from build123d import *

# Parameters (mm, degrees)
EXT_LUG_DEPTH = 2.4892


with BuildPart() as part:
    # Sk_kingpin_section → Rev_kingpin (revolve)
    with BuildSketch(Plane.XY, mode=Mode.PRIVATE) as rev_kingpin_sk:
        with BuildLine():
            Line((0, 54.2544), (5.9944, 52.64912))
            Line((5.9944, 52.64912), (5.9944, 45.12818))
            Line((5.9944, 45.12818), (6.49478, 44.6278))
            Line((6.49478, 44.6278), (6.93928, 44.6278))
            Line((6.93928, 44.6278), (7.43839, 45.12818))
            Line((7.43839, 45.12818), (7.43839, 60.1218))
            ThreePointArc((7.43839, 60.1218), (7.549982316, 60.391207684), (7.81939, 60.5028))
            Line((7.81939, 60.5028), (9.1567, 60.5028))
            ThreePointArc((9.1567, 60.5028), (9.426107684, 60.614392316), (9.5377, 60.8838))
            Line((9.5377, 60.8838), (9.5377, 63.1698))
            ThreePointArc((9.5377, 63.1698), (9.426107684, 63.439207684), (9.1567, 63.5508))
            Line((9.1567, 63.5508), (7.9121, 63.5508))
            ThreePointArc((7.9121, 63.5508), (7.642692316, 63.662392316), (7.5311, 63.9318))
            Line((7.5311, 63.9318), (7.5311, 69.34962))
            Line((7.5311, 69.34962), (7.03072, 69.85))
            Line((7.03072, 69.85), (0, 69.85))
            Line((0, 69.85), (0, 54.2544))
        make_face()
    revolve(rev_kingpin_sk.sketch.rotate(Axis((0, -25.4, 0), (0, 1, 0)), 90), axis=Axis((0, -25.4, 0), (0, 1, 0)))

    # Sk_lug → Ext_lug (add)
    with BuildSketch(Plane(origin=(0, 63.5508, 0), x_dir=(1, 0, 0), z_dir=(0, 1, 0))):
        with BuildLine():
            Line((-7.19328, 2.23012), (-7.19328, -2.23012))
            ThreePointArc((-7.19328, -2.23012), (-7.46394509, -1.797883422), (-7.9121, -1.55448))
            ThreePointArc((-7.9121, -1.55448), (-9.1313, 0), (-7.9121, 1.55448))
            ThreePointArc((-7.9121, 1.55448), (-7.463342343, 1.797242155), (-7.19328, 2.23012))
        make_face()
    extrude(amount=EXT_LUG_DEPTH)


solid = part.part
Can you work these out from the model? Positions are in its coordinate system, mm. A direction names the side the tool comes from. Give positions to 0.01 mm unless a question says otherwise; leave off trailing zeros. Order: outer loops, then holes, each group sorted by start corner. A loop starts at its lowest first (then second) coordinate and runs counter-clockwise, first axis right, second up. Notation, with made-up numbers: M 45,-14.75 L 60,-14.75 A23 cw 60,20.25 Z; hole C 73,62 d7. An arc over 180 degrees is marked long. Use a Markdown table: item, result. Add a question column.
Item 1: We'd pull the mould along Z, two halves only. Please class faces 6 (the flat face through (0, 69.85, 0)), 7 (the conical face through (0.366, 54.154, 0.081)), 8 (the cylindrical face through (7.352, 66.679, 1.633)): +Z half, -Z half, draft (parallel to the pull), parting line (faces both ways), or undercut.
Item 2: Will these pins go through, and if not, where does the flat tip stop? pin 1 (8 mm diameter, centred on x = 4.5, y = 58.5, fed in from -Z); pin 2 (5 mm diameter, centred on y = 63.5, z = -6.5, fed in from +X); pin 3 (4 mm diameter, centred on y = 47.5, z = 4.5, fed in from -X); pin 4 (8 mm diameter, centred on x = -1, z = 4.5, fed in from -Y).
Item 3: If I drill on L1, parallel to X at y = 49.75, z = 0; L2, parallel to X at y = 49, z = -3.5; L3, parallel to Y at x = -8.5, z = -3.25, over which ranges is the centre line in solid material (lowest first)? Write a range as [from, to].
Item 4: Suppose I cut it at A-A (y = 57.25). List the corners of the cut face in (x, z) for me, then the cut area to 3 significant figures.
Item 5: For faces 1 (the cylindrical face through (-9.13, 64.78, 0.03)), 2 (the flat face through (8.1, 63.551, 0)), 3 (the cylindrical face through (5.8, 62.04, 7.57)), 4 (the cylindrical face through (-1.801, 48.836, -5.718)), 5 (the flat face through (3, 44.628, 6)), which set-ups out of +Z, -Z, +X, -X, +Y, -Y let a thin tool reach every point of the face, with its end or its side?
Answer sheet:
| question | item | result |
|---|---|---|
| 1 | face 6 | draft |
| 1 | face 7 | undercut |
| 1 | face 8 | parting line |
| 2 | pin 1 | stops at z = -9.45 |
| 2 | pin 2 | stops at x = 8.65 |
| 2 | pin 3 | stops at x = -7.01 |
| 2 | pin 4 | stops at y = 44.63 |
| 3 | L1 | x = [-7.44, -5.99], [5.99, 7.44] |
| 3 | L2 | x = [-6.56, -4.87], [4.87, 6.56] |
| 3 | L3 | y = [60.5, 63.55] |
| 4 | outline | C 0,0 d14.88 |
| 4 | area | 174 mm² |
| 5 | face 1 | -X, +Y |
| 5 | face 2 | +Y |
| 5 | face 3 | +Y, -Y |
| 5 | face 4 | -Y |
| 5 | face 5 | +Z, -Z, +X, -X, -Y |
